The model under review builds one solid part; all positions refer to its coordinate system, in mm. Give positions to 0.01 mm unless a question says otherwise; leave off trailing zeros. Loops run counter-clockwise (first coordinate to the right, second up) from the corner with the lowest first, then second, coordinate; pieces in that order, holes last. Notation, with made-up numbers: M 16,13 L 57,13 A16 cw 57,18 Z; hole C -37.75,57.25 d5. An arc over 180 degrees is marked long. Write item = value, one per line. Start each with the question number.
1. We need section B-B on z = 881. Give the boundary of the cut face in (x, y).
2. We need section A-A on y = 9.75. Give the boundary of the cut face in (x, z), then the cut area to 3 significant figures.
3. We need section C-C on x = 22.5. Give the boundary of the cut face in (y, z), then the cut area to 3 significant figures.
4. Wall thickness on line 1 along X through (y, z) = (0.7, 438); line 2 along X through (y, z) = (10.25, 527.5); line 3 along Y through (x, z) = (8, 526.5): over which ranges is each line inside the solid? List them lowest first. Write a range as from..to.
5. Draft analysis for pull direction Y (two halves, no side actions). For faces 1 (the face through (20, 14, 493)), 2 (the face through (20, 15, 493)), 3 (the face through (20, 0, 493)), state which applies: pulls with the +Y half, pulls with the -Y half, needs draft (parallel to the pull), parting line crosses it, or undercut.
from build123d import *

# Parameters (mm, degrees)
SKETCH_1_W          = 40
SKETCH_1_H          = 15
SKETCH_1_W_2        = 38
SKETCH_1_H_2        = 13
EXTRUDE_1_DEPTH     = 1000
SKETCH_3_R          = 2.5
CUT_EXTRUDE_2_DEPTH = 1001.912084051


with BuildPart() as part:
    # 草图1 → 凸台-拉伸1 (new body)
    with BuildSketch(Plane.XY):
        with Locations((20, 7.5)):
            Rectangle(SKETCH_1_W, SKETCH_1_H)
        with Locations((20, 7.5)):
            Rectangle(SKETCH_1_W_2, SKETCH_1_H_2, mode=Mode.SUBTRACT)
    extrude(amount=EXTRUDE_1_DEPTH)

    # 草图3 → 切除-拉伸2 (cut, through all)
    with BuildSketch(Plane.XZ):
        with Locations(Location((35, 468, 0), (0, 0, 270))):
            Circle(SKETCH_3_R)
        with Locations(Location((35, 438, 0), (0, 0, 270))):
            Circle(SKETCH_3_R)
        with Locations(Location((5, 468, 0), (0, 0, 270))):
            Circle(SKETCH_3_R)
        with Locations(Location((5, 438, 0), (0, 0, 270))):
            Circle(SKETCH_3_R)
    extrude(amount=-CUT_EXTRUDE_2_DEPTH, mode=Mode.SUBTRACT)


solid = part.part
Final values:
q1.outline = M 0,0 L 40,0 L 40,15 L 0,15 Z; hole M 1,1 L 39,1 L 39,14 L 1,14 Z
q2.outline = M 0,0 L 1,0 L 1,1000 L 0,1000 Z; M 39,0 L 40,0 L 40,1000 L 39,1000 Z
q2.area = 2,000 mm²
q3.outline = M 0,0 L 1,0 L 1,1000 L 0,1000 Z; M 14,0 L 15,0 L 15,1000 L 14,1000 Z
q3.area = 2,000 mm²
q4.line_1 = 0..2.5, 7.5..32.5, 37.5..40
q4.line_2 = 0..1, 39..40
q4.line_3 = 0..1, 14..15
q5.face_1 = undercut
q5.face_2 = pulls with the +Y half
q5.face_3 = pulls with the -Y half
